Here's how the part is built. I have some questions about the finished solid (model axes, mm). A direction names the side the tool comes from. Round coordinates to 2 decimals unless told otherwise and drop trailing zeros. Loops run counter-clockwise (first coordinate to the right, second up) from the corner with the lowest first, then second, coordinate; pieces in that order, holes last. Notation, with made-up numbers: (62.25, -18) - (99.25, -18) arc R20 cw to (99.25, 3) - close; hole circle Ø6 at (-30.5, 30). An arc over 180 degrees is marked (long way). Return JSON: item names as keys, results as strings. Group by question number.
Autodesk Fusion 360 part; units mm, degrees
sketch "Sketch1" plane through (0, 0, 0) normal (0, 0, 1) x (1, 0, 0)
  line L0 (16, 15) -> (-16, 15)
  line L1 (-16, 15) -> (-16, -15)
  line L2 (-16, -15) -> (16, -15)
  line L3 (16, -15) -> (16, 15)
  line L4 (-16, 15) -> (16, -15) construction
  line L5 (14, 10.25) -> (-14, -10.25) construction
  line L6 (-14.6684, 10.7394) -> (14, -10.25) construction
  line L7 (14, -10.25) -> (14, 10.75)
  line L8 (14, 10.75) -> (-14, 10.75)
  line L9 (-14, 10.75) -> (-14, -10.25)
  line L10 (-14, -10.25) -> (14, -10.25)
  dimension "d1" = 32
  dimension "d2" = 30
  dimension "d3" = 28
  dimension "d4" = 21
  dimension "d33" = 28
  dimension "d34" = 21
extrude "Extrude1" add sketch "Sketch1" along normal blind 6 contours L0 L1 L2 L3 | L7 L8 L9 L10
sketch "Sketch2" plane through (0, 0, 6) normal (0, 0, 1) x (-1, 0, 0)
  line L0 (-16, 15) -> (-16, -15)
  line L1 (-16, -15) -> (16, -15)
  line L2 (16, -15) -> (16, 15)
  line L3 (16, 15) -> (-16, 15)
  line L4 (6.895, -15) -> (-6.895, -15)
  line L5 (-6.895, -15) -> (-6.895, -11.3)
  line L6 (-6.895, -11.3) -> (6.895, -11.3)
  line L7 (6.895, -11.3) -> (6.895, -15)
  dimension "d7" = 13.79
  dimension "d8" = 3.7
extrude "Extrude2" cut sketch "Sketch2" against normal blind 5 contours L1 L4 L5 L6 L7
sketch "Sketch3" plane through (0, 0, 6) normal (0, 0, 1) x (-1, 0, 0)
  line L0 (6.895, -11.3) -> (6.895, -15)
  line L1 (6.895, -15) -> (16, -15)
  line L2 (16, -15) -> (16, 15)
  line L3 (16, 15) -> (-16, 15)
  line L4 (-16, 15) -> (-16, -15)
  line L5 (-16, -15) -> (-6.895, -15)
  line L6 (-6.895, -15) -> (-6.895, -11.3)
  line L7 (-6.895, -11.3) -> (6.895, -11.3)
  line L8 (-13.75, -13.75) -> (13.75, -13.75)
  line L9 (13.75, -13.75) -> (13.75, 13.75)
  line L10 (13.75, 13.75) -> (-13.75, 13.75)
  line L11 (-13.75, 13.75) -> (-13.75, -13.75)
  line L12 (-13.75, -13.75) -> (13.75, 13.75) construction
  line L13 (13.75, -13.75) -> (-13.75, 13.75) construction
  line L14 (-13.75, -13.75) -> (-12.25, -13.75)
  line L15 (-13.75, -12.25) -> (-13.75, -13.75)
  circle A0 centre (-12.25, -12.25) radius 0.85
  line L16 (13.75, -13.75) -> (11.25, -13.75)
  line L17 (13.75, -12.25) -> (13.75, -13.75)
  circle A1 centre (11.25, -12.25) radius 0.85
  line L18 (13.75, 13.75) -> (11.25, 13.75)
  line L19 (13.75, 11.25) -> (13.75, 13.75)
  circle A2 centre (11.75, 11.25) radius 0.85
  line L20 (-13.75, 13.75) -> (-12.25, 13.75)
  line L21 (-13.75, 12.25) -> (-13.75, 13.75)
  circle A3 centre (-11.75, 11.25) radius 0.85
  line L22 (8.2149, 11.25) -> (8.2149, 11.2573)
  line L23 (-13.75, 13.75) -> (-11.25, 13.75)
  line L24 (-13.75, 11.25) -> (-13.75, 13.75)
  line L25 (-13.75, -13.75) -> (-12.25, -13.75)
  line L26 (-13.75, -11.25) -> (-13.75, -13.75)
  line L27 (13.75, -13.75) -> (11.25, -13.75)
  line L28 (13.75, -11.25) -> (13.75, -13.75)
  line L29 (11.25, -12.25) -> (-12.25, -12.25)
  line L30 (-11.75, 11.25) -> (11.75, 11.25)
  dimension "d11" = 27.5
  dimension "d12" = 27.5
  dimension "d15" = 1.7
  dimension "d18" = 1.7
  dimension "d19" = 2.5
  dimension "d20" = 2.5
  dimension "d21" = 1.7
  dimension "d22" = 1.5
  dimension "d23" = 1.5
  dimension "d24" = 1.7
  dimension "d27" = 2.5
  dimension "d28" = 2.5
  dimension "d30" = 2.5
  dimension "d31" = 2.5
  dimension "d32" = 2.5
  dimension "d37" = 23.5
  dimension "d38" = 23.5
extrude "Extrude3" cut sketch "Sketch3" against normal blind 5 contours A1 | A0 | A2 | A3
extrude "Extrude4" cut sketch "Sketch1" along normal blind 6 contours L7 L8 L9 L10
Q1. Will these pins go through, and if not, where does the flat tip stop? pin 1 Ø1.5 at (x, y) = (-11.75, -11.25) entering from +Z; pin 2 Ø3 at (x, z) = (4, 4) entering from +Y.
Q2. Imagine slicing it at D-D, the plane y = -11.25. List the corners of the cut face in (x, z) for me.
Q3. Imagine slicing it at B-B, the plane y = 3.5. List the corners of the cut face in (x, z) for me.
Q4. Imagine slicing it at A-A, the plane x = 2.5. List the corners of the cut face in (y, z) for me, and give its area (3 significant figures).
Q5. Please list where these lines run through material, in increasing order: line 1 (X direction, y = -11.25, z = 4.9); line 2 (X direction, y = 12.25, z = 4.55) (3 decimals); line 3 (X direction, y = -7.25, z = 4.6).
Q6. Imagine slicing it at C-C, the plane z = 4.9. List the corners of the cut face in (x, y) for me (3 decimals), and give its area (3 significant figures).
Q7. For faces 4 (the flat face through (0, 13, 1)), 5 (the flat face through (0, -15, 3)), 6 (the cylindrical face through (11.793, 11.533, 3.535)), 7 (the flat face through (0.2, 15, 0.3)), 8 (the flat face through (-14, 0, 3)), which set-ups out of +Z, -Z, +X, -X, +Y, -Y let a thin tool reach every point of the face, with its end or its side?
Q8. If we mould it in two halves opening along X, with no side actions, what happens to faces 1 (the flat face through (12, -11, 1)), 2 (the flat face through (-16, 0, 3)), 3 (the flat face through (0, -11, 6))? For each: +X half, -X half, draft (parallel to the pull), parting line (faces both ways), or undercut.
Output values:
{
 "1": {"pin 1": "stops at z = 1", "pin 2": "stops at y = 11.3"},
 "2": {"outline": "(-16, 0) - (16, 0) - (16, 6) - (12.6, 6) - (12.6, 1) - (10.9, 1) - (10.9, 6) - (-10.9, 6) - (-10.9, 1) - (-12.6, 1) - (-12.6, 6) - (-16, 6) - close"},
 "3": {"outline": "(-16, 0) - (-14, 0) - (-14, 6) - (-16, 6) - close; (14, 0) - (16, 0) - (16, 6) - (14, 6) - close"},
 "4": {"outline": "(-15, 0) - (-10.25, 0) - (-10.25, 6) - (-15, 6) - close; (10.75, 0) - (15, 0) - (15, 1) - (11.3, 1) - (11.3, 6) - (10.75, 6) - close", "area": "35.5 mm^2"},
 "5": {"line 1": "x = -16 to -12.6, -10.9 to 10.9, 12.6 to 16", "line 2": "x = -16 to -12.1, -10.4 to -6.895, 6.895 to 11.4, 13.1 to 16", "line 3": "x = -16 to -14, 14 to 16"},
 "6": {"outline": "(-16, -15) - (16, -15) - (16, 15) - (6.895, 15) - (6.895, 11.3) - (-6.895, 11.3) - (-6.895, 15) - (-16, 15) - close; hole (-14, -10.25) - (14, -10.25) - (14, 10.75) - (-14, 10.75) - close; hole circle Ø1.7 at (-11.75, -11.25); hole circle Ø1.7 at (-11.25, 12.25); hole circle Ø1.7 at (11.75, -11.25); hole circle Ø1.7 at (12.25, 12.25)", "area": "312 mm^2"},
 "7": {"face 4": "+Z, +Y", "face 5": "+Z, -Z, +X, -X, -Y", "face 6": "+Z", "face 7": "+Z, -Z, +X, -X, +Y", "face 8": "+Z, -Z"},
 "8": {"face 1": "undercut", "face 2": "-X half", "face 3": "draft"}
}
